Design review of the part built by this model. Coordinates are the model's own, in mm. Face numbers are marked on the shaded views. A direction names the side the tool comes from. Give positions to 0.01 mm unless a question says otherwise; leave off trailing zeros. Write each loop counter-clockwise with the first axis right and the second up, starting at its lowest first coordinate (ties: lowest second). Pieces come first, ordered by that corner, then holes. Notation, with made-up numbers: (13, -35) -> (66, -35) arc R27 ccw to (66, -13) -> close; hole circle Ø1 at (0.5, -24). An arc over 180 degrees is marked (long way). Answer as a JSON object with one key per item and string values.
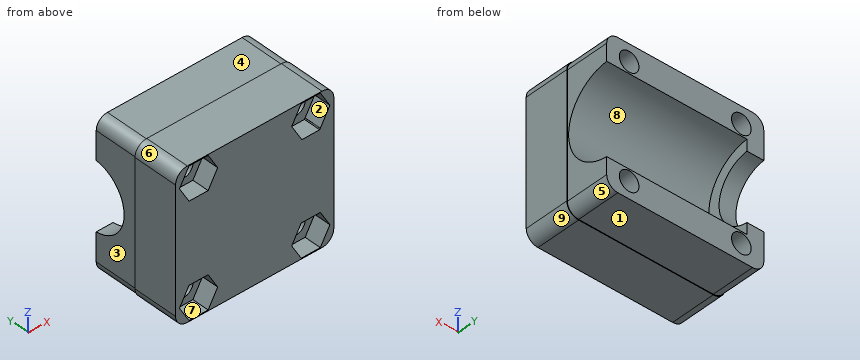
```python
from build123d import *

# Parameters (mm, degrees)
SKETCH1_W           = 26
SKETCH1_H           = 32.5
SKETCH1_R           = 8
BOSS_EXTRUDE1_DEPTH = 14
SKETCH2_R           = 1.75
CUT_EXTRUDE1_DEPTH  = 72
SKETCH3_W           = 26
SKETCH3_H           = 16.75
CUT_EXTRUDE3_DEPTH  = 32
FILLET2_R           = 2
BOSS_EXTRUDE2_DEPTH = 3
CUT_EXTRUDE4_DEPTH  = 3
BOSS_EXTRUDE3_DEPTH = 8
CUT_EXTRUDE5_DEPTH  = 3
CUT_EXTRUDE6_DEPTH  = 25.010414407


with BuildPart() as part:
    # Sketch1 → Boss-Extrude1 (new, symmetric)
    with BuildSketch(Plane(origin=(0, 0, 0), x_dir=(0, 0, -1), z_dir=(1, 0, 0))):
        Rectangle(SKETCH1_W, SKETCH1_H)
        Circle(SKETCH1_R, mode=Mode.SUBTRACT)
    extrude(amount=BOSS_EXTRUDE1_DEPTH, both=True)

    # Sketch2 → Cut-Extrude1 (cut)
    with BuildSketch(Plane(origin=(0, 16.25, 0), x_dir=(1, 0, 0), z_dir=(0, 1, 0))):
        with Locations(Location((-10, 10, 0), (0, 0, 270))):
            Circle(SKETCH2_R)
        with Locations(Location((10, 10, 0), (0, 0, 270))):
            Circle(SKETCH2_R)
        with Locations(Location((10, -10, 0), (0, 0, 270))):
            Circle(SKETCH2_R)
        with Locations(Location((-10, -10, 0), (0, 0, 270))):
            Circle(SKETCH2_R)
    extrude(amount=-CUT_EXTRUDE1_DEPTH, mode=Mode.SUBTRACT)

    # Sketch3 → Cut-Extrude3 (cut)
    with BuildSketch(Plane.ZY.offset(14)):
        with Locations((0, 7.875)):
            Rectangle(SKETCH3_W, SKETCH3_H)
    extrude(amount=-CUT_EXTRUDE3_DEPTH, mode=Mode.SUBTRACT)

    # Fillet2
    fillet2_edges = [part.edges().sort_by_distance(p)[0] for p in [
        (-14, -8.375, 13),
        (14, -8.375, 13),
        (14, -8.375, -13),
        (-14, -8.375, -13),
    ]]
    fillet(fillet2_edges, radius=FILLET2_R)

    # Sketch4 → Boss-Extrude2 (add)
    with BuildSketch(Plane(origin=(-14, 0, 0), x_dir=(0, 0, -1), z_dir=(1, 0, 0))):
        with BuildLine():
            Line((-7.984359711, -0.5), (-5.979130372, -0.5))
            ThreePointArc((-5.979130372, -0.5), (0, -6), (5.979130372, -0.5))
            Line((5.979130372, -0.5), (7.984359711, -0.5))
            ThreePointArc((7.984359711, -0.5), (0, -8), (-7.984359711, -0.5))
        make_face()
    extrude(amount=BOSS_EXTRUDE2_DEPTH)

    # Sketch5 → Cut-Extrude4 (cut)
    with BuildSketch(Plane.XZ.offset(16.25)):
        Polygon((-6.593633412, 10), (-8.296816706, 12.95), (-11.703183294, 12.95), (-13.406366588, 10), (-11.703183294, 7.05), (-8.296816706, 7.05), align=None)
        Polygon((8.41228676, 6.85), (6.824573519, 10), (8.41228676, 12.75), (11.58771324, 12.75), (13.175426481, 10), (11.58771324, 6.85), align=None)
        Polygon((6.824573519, -10), (8.41228676, -12.75), (11.58771324, -12.75), (13.175426481, -10), (11.58771324, -7.25), (8.41228676, -7.25), align=None)
        Polygon((-8.41228676, -7.25), (-6.824573519, -10), (-8.41228676, -12.75), (-11.58771324, -12.75), (-13.175426481, -10), (-11.58771324, -7.25), align=None)
    extrude(amount=-CUT_EXTRUDE4_DEPTH, mode=Mode.SUBTRACT)

    # Sketch6 → Boss-Extrude3 (add)
    with BuildSketch(Plane.XZ.offset(16.25)):
        with BuildLine():
            Line((-12, -15.5), (12, -15.5))
            ThreePointArc((12, -15.5), (15.181980515, -14.181980515), (16.5, -11))
            Line((16.5, -11), (16.5, 11))
            ThreePointArc((16.5, 11), (15.181980515, 14.181980515), (12, 15.5))
            Line((12, 15.5), (-12, 15.5))
            ThreePointArc((-12, 15.5), (-15.181980515, 14.181980515), (-16.5, 11))
            Line((-16.5, 11), (-16.5, -11))
            ThreePointArc((-16.5, -11), (-15.181980515, -14.181980515), (-12, -15.5))
        make_face()
        with BuildLine():
            Line((-12, -13), (12, -13))
            ThreePointArc((12, -13), (13.414213562, -12.414213562), (14, -11))
            Line((14, -11), (14, 11))
            ThreePointArc((14, 11), (13.414213562, 12.414213562), (12, 13))
            Line((12, 13), (-12, 13))
            ThreePointArc((-12, 13), (-13.414213562, 12.414213562), (-14, 11))
            Line((-14, 11), (-14, -11))
            ThreePointArc((-14, -11), (-13.414213562, -12.414213562), (-12, -13))
        make_face(mode=Mode.SUBTRACT)
    extrude(amount=-BOSS_EXTRUDE3_DEPTH)

    # Sketch7 → Cut-Extrude5 (cut)
    with BuildSketch(Plane.XZ.offset(16.25)):
        Polygon((-6.593633412, 10), (-8.296816706, 12.95), (-11.703183294, 12.95), (-13.406366588, 10), (-11.703183294, 7.05), (-8.296816706, 7.05), align=None)
        Polygon((13.406366588, 10), (11.703183294, 12.95), (8.296816706, 12.95), (6.593633412, 10), (8.296816706, 7.05), (11.703183294, 7.05), align=None)
        Polygon((-6.593633412, -10), (-8.296816706, -7.05), (-11.703183294, -7.05), (-13.406366588, -10), (-11.703183294, -12.95), (-8.296816706, -12.95), align=None)
        Polygon((13.406366588, -10), (11.703183294, -7.05), (8.296816706, -7.05), (6.593633412, -10), (8.296816706, -12.95), (11.703183294, -12.95), align=None)
    extrude(amount=-CUT_EXTRUDE5_DEPTH, mode=Mode.SUBTRACT)

    # Sketch8 → Cut-Extrude6 (cut, through all)
    with BuildSketch(Plane(origin=(0, -8.25, 0), x_dir=(1, 0, 0), z_dir=(0, 1, 0))):
        with BuildLine():
            Line((-12, -15.7), (12, -15.7))
            ThreePointArc((12, -15.7), (15.323401872, -14.323401872), (16.7, -11))
            Line((16.7, -11), (16.7, 11))
            ThreePointArc((16.7, 11), (15.323401872, 14.323401872), (12, 15.7))
            Line((12, 15.7), (-12, 15.7))
            ThreePointArc((-12, 15.7), (-15.323401872, 14.323401872), (-16.7, 11))
            Line((-16.7, 11), (-16.7, -11))
            ThreePointArc((-16.7, -11), (-15.323401872, -14.323401872), (-12, -15.7))
        make_face()
        with BuildLine():
            Line((-14.1, 11), (-14.1, -11))
            ThreePointArc((-14.1, -11), (-13.48492424, -12.48492424), (-12, -13.1))
            Line((-12, -13.1), (12, -13.1))
            ThreePointArc((12, -13.1), (13.48492424, -12.48492424), (14.1, -11))
            Line((14.1, -11), (14.1, 11))
            ThreePointArc((14.1, 11), (13.48492424, 12.48492424), (12, 13.1))
            Line((12, 13.1), (-12, 13.1))
            ThreePointArc((-12, 13.1), (-13.48492424, 12.48492424), (-14.1, 11))
        make_face(mode=Mode.SUBTRACT)
    extrude(amount=-CUT_EXTRUDE6_DEPTH, mode=Mode.SUBTRACT)


solid = part.part
```
(1) For line 1 along X through (y, z) = (-4.75, 10); line 2 along X through (y, z) = (-15.25, 7.75); line 3 along Z through (x, y) = (9.5, -12), list the stretches that pass through material, from the lowest coordinate up.
Here are the results:
{"line 1": "x = -14 to -11.75, -8.25 to 8.25, 11.75 to 14", "line 2": "x = -14.1 to -12.11, -7.89 to 7.89, 12.11 to 14.1", "line 3": "z = -13.1 to -11.68, -8.32 to 8.32, 11.68 to 13.1"}
(2) For the marked faces 1, 2, 3, 4 and 5, list the 3-axis set-ups (+Z, -Z, +X, -X, +Y, -Y) from which the entire face can be reached by the end or side of a thin tool; tool diameter is ignored.
Here are the results:
{"face 1": "-Z, +X, -X, +Y", "face 2": "-Y", "face 3": "+Z, -Z, -X, +Y", "face 4": "+Z, +X, -X, +Y", "face 5": "-Z, +X, +Y"}
(3) We need section A-A, the plane x = -10. State the section outline as (y, z) points, then the cut area to 3 significant figures.
Here are the results:
{"outline": "(-16.25, -13.1) -> (-8.25, -13.1) -> (-8.25, -13) -> (-0.5, -13) -> (-0.5, -11.75) -> (-13.25, -11.75) -> (-13.25, -12.95) -> (-16.25, -12.95) -> close; (-16.25, -7.05) -> (-13.25, -7.05) -> (-13.25, -8.25) -> (-0.5, -8.25) -> (-0.5, -7.98) arc R8 cw to (-0.5, 7.98) -> (-0.5, 8.25) -> (-13.25, 8.25) -> (-13.25, 7.05) -> (-16.25, 7.05) -> close; (-16.25, 12.95) -> (-13.25, 12.95) -> (-13.25, 11.75) -> (-0.5, 11.75) -> (-0.5, 13) -> (-8.25, 13) -> (-8.25, 13.1) -> (-16.25, 13.1) -> close", "area": "194 mm²"}
(4) The part is to be moulded in two halves that separate along X. For the marked faces 6, 7, 8 and 9, say which applies: +X half, -X half, draft (parallel to the pull), parting line (faces both ways), or undercut.
Here are the results:
{"face 6": "-X half", "face 7": "undercut", "face 8": "draft", "face 9": "+X half"}
(5) We need section C-C, the plane z = 0. State the section outline as (x, y) points, then the cut area to 3 significant figures.
Here are the results:
{"outline": "(-14.1, -16.25) -> (14.1, -16.25) -> (14.1, -8.25) -> (14, -8.25) -> (14, -8) -> (-11, -8) -> (-11, -6) -> (-14, -6) -> (-14, -8.25) -> (-14.1, -8.25) -> close", "area": "239 mm²"}
(6) We need section B-B, the plane y = -2.5. State the section outline as (x, z) points, then the cut area to 3 significant figures.
Here are the results:
{"outline": "(-14, -11) arc R2 ccw to (-12, -13) -> (12, -13) arc R2 ccw to (14, -11) -> (14, -7.6) -> (-11, -7.6) -> (-11, -5.45) -> (-14, -5.45) -> close; (-14, 5.45) -> (-11, 5.45) -> (-11, 7.6) -> (14, 7.6) -> (14, 11) arc R2 ccw to (12, 13) -> (-12, 13) arc R2 ccw to (-14, 11) -> close; hole circle Ø3.5 at (-10, -10); hole circle Ø3.5 at (-10, 10); hole circle Ø3.5 at (10, -10); hole circle Ø3.5 at (10, 10)", "area": "273 mm²"}
(7) Clearance check with flat-ended pins moving along their axes: pin 1 (2 mm diameter, centred on x = -9.5, z = -9, fed in from -Y); pin 2 (1.5 mm diameter, centred on x = -7, z = -0.5, fed in from +Y); pin 3 (1.5 mm diameter, centred on x = 5, z = 3, fed in from +Y). State where each tip first meets the part, or that it passes through.
Here are the results:
{"pin 1": "stops at y = -13.25", "pin 2": "stops at y = -7.9", "pin 3": "stops at y = -7.07"}
(8) We need section D-D, the plane y = -10.75. State the section outline as (x, z) points.
Here are the results:
{"outline": "(-14.1, -11) arc R2.1 ccw to (-12, -13.1) -> (12, -13.1) arc R2.1 ccw to (14.1, -11) -> (14.1, 11) arc R2.1 ccw to (12, 13.1) -> (-12, 13.1) arc R2.1 ccw to (-14.1, 11) -> close; hole circle Ø3.5 at (-10, -10); hole circle Ø3.5 at (-10, 10); hole circle Ø3.5 at (10, -10); hole circle Ø3.5 at (10, 10)"}
